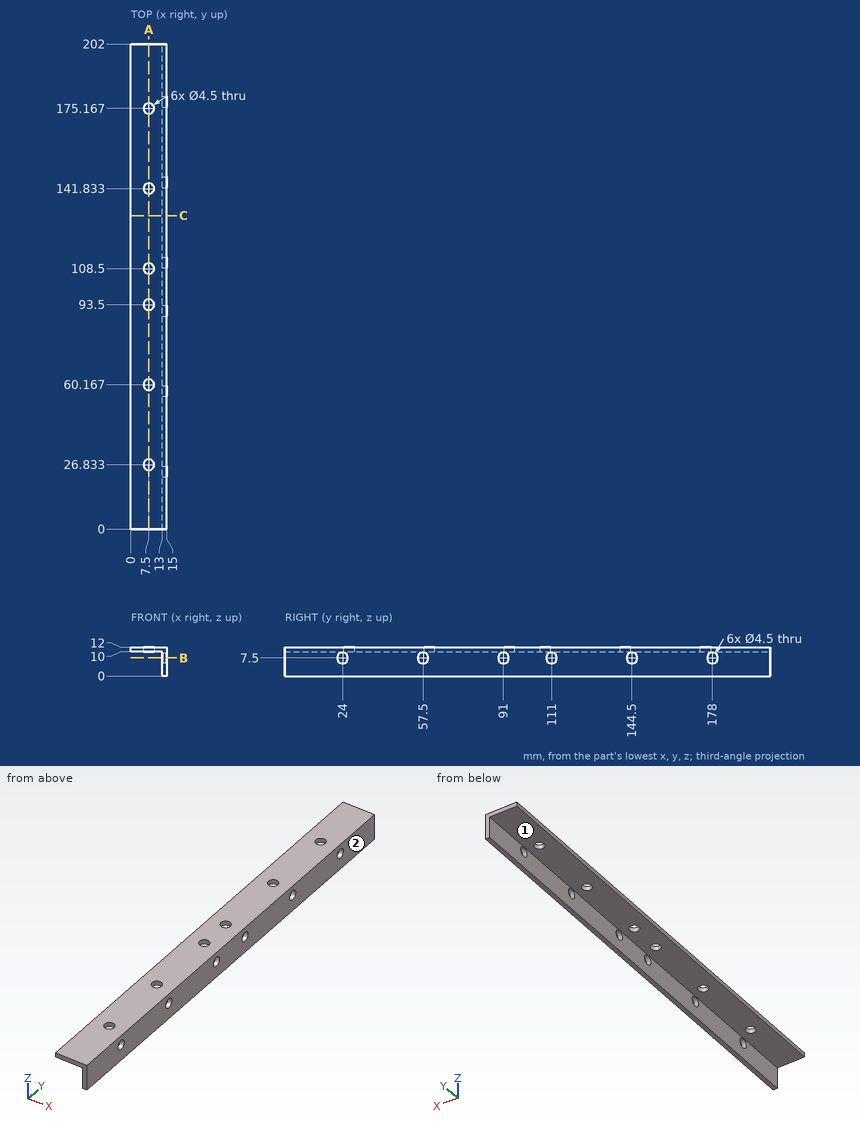
Can you work these out from the drawing? Everything is in mm from the part's minimum corner. A direction names the side the tool comes from. Give positions to 0.01 mm unless a question says otherwise; leave off trailing zeros. Loops run counter-clockwise (first coordinate to the right, second up) from the corner with the lowest first, then second, coordinate; pieces in that order, holes last. Notation, with made-up numbers: M 86.25,13 L 139.25,13 A34 ccw 139.25,51 Z; hole C 49.5,-20 d5. An arc over 180 degrees is marked long. Put each result on its own line as item: value. Start each with the question number.
(1) I want a section at A-A on x = 7.5. Please give me the cut outline in (y, z).
(2) For the marked faces 1 and 2, which set-ups out of +Z, -Z, +X, -X, +Y, -Y let a thin tool reach every point of the face, with its end or its side?
(3) I want a section at B-B on z = 7.5. Please give me the cut outline in (x, y), then the cut area to 3 significant figures.
(4) Will these pins go through, and if not, where does the flat tip stop? pin 1 Ø1.5 at (x, y) = (11.5, 50) entering from -Z; pin 2 Ø1.5 at (y, z) = (151.5, 3) entering from -X; pin 3 Ø2.5 at (x, y) = (7.5, 26.83) entering from -Z; pin 4 Ø7 at (y, z) = (144.5, 7.5) entering from +X.
(5) I need wall thicknesses on line 1 along Z through (x, y) = (13.55, 144.5); line 2 along Z through (x, y) = (7, 66.5); line 3 along X through (y, z) = (51.5, 1.25). Which ranges of each line are inside material? Lowest first, please. Write a range as [from, to].
(6) I want a section at C-C on y = 130.5. Please give me the cut outline in (x, z), then the cut area to 3 significant figures.
Answer block:
1. outline: M 0,10 L 24.58,10 L 24.58,12 L 0,12 Z; M 29.08,10 L 57.92,10 L 57.92,12 L 29.08,12 Z; M 62.42,10 L 91.25,10 L 91.25,12 L 62.42,12 Z; M 95.75,10 L 106.25,10 L 106.25,12 L 95.75,12 Z; M 110.75,10 L 139.58,10 L 139.58,12 L 110.75,12 Z; M 144.08,10 L 172.92,10 L 172.92,12 L 144.08,12 Z; M 177.42,10 L 202,10 L 202,12 L 177.42,12 Z
2. face 1: -Z, -X, +Y, -Y
2. face 2: +Z, -Z, +X, +Y, -Y
3. outline: M 13,0 L 15,0 L 15,21.75 L 13,21.75 Z; M 13,26.25 L 15,26.25 L 15,55.25 L 13,55.25 Z; M 13,59.75 L 15,59.75 L 15,88.75 L 13,88.75 Z; M 13,93.25 L 15,93.25 L 15,108.75 L 13,108.75 Z; M 13,113.25 L 15,113.25 L 15,142.25 L 13,142.25 Z; M 13,146.75 L 15,146.75 L 15,175.75 L 13,175.75 Z; M 13,180.25 L 15,180.25 L 15,202 L 13,202 Z
3. area: 350 mm^2
4. pin 1: z = 10
4. pin 2: x = 13
4. pin 3: through
4. pin 4: x = 15
5. line 1: [0, 5.25], [9.75, 12]
5. line 2: [10, 12]
5. line 3: [13, 15]
6. outline: M 0,10 L 13,10 L 13,0 L 15,0 L 15,12 L 0,12 Z
6. area: 50.0 mm^2
